Could you check a few things on this model? Use its own coordinates, in mm. Face numbers are marked on the shaded views. A direction names the side the tool comes from. Round coordinates to 2 decimals unless told otherwise and drop trailing zeros. Write each loop counter-clockwise with the first axis right and the second up, starting at its lowest first coordinate (ties: lowest second). Pieces come first, ordered by that corner, then holes. Notation, with made-up numbers: M 3,33 L 23,33 A9 ccw 23,50 Z; hole C 71,12 d11. An arc over 180 degrees is marked long. One line per item, written item: value. Start each with the question number.
(1) If I drill on L1, parallel to X at y = -20, z = 8; L2, parallel to Y at x = 24, z = 6; L3, parallel to X at y = 5, z = 6.5, over which ranges is the centre line in solid material (lowest first)?
(2) Which directions (+Z, -Z, +X, -X, +Y, -Y) give clear straight access to the entire face, cutting with the end or side of a thin tool? Please do the marked faces 5 and 6.
(3) I want a section at B-B on z = 6.5. Please give me the cut outline in (x, y), and give its area (3 significant figures).
(4) I'm going to push a flat-ended pin straight in: pin 1 Ø23.5 at (x, y) = (14, -3) entering from +Z. Where does the tip first touch, or does it pass through?
(5) Thinking about a two-plate mould opening in X: for the marked faces 1, 2, 3 and 4, which applies, released by +X, released by -X, zero draft, split by the parting line, or undercut?
```python
from build123d import *

# Parameters (mm, degrees)
F0_W     = 117.221
F0_H     = 53.721
F1_DEPTH = 19.05
F2_R     = 3.175
F3_T     = -2.54
F5_W     = 11.2527239306
F5_H     = 9.8262102796
F5_W_2   = 11.6953600091
F5_H_2   = 12.192
F6_DEPTH = 17.78


# Not quite as in the source:
# - a feature names something its author has since deleted; it is built from what else it names


with BuildPart() as f1:
    # F0 (on Top) → F1 (new body)
    with BuildSketch(Plane.XY):
        Rectangle(F0_W, F0_H)
    extrude(amount=F1_DEPTH)

    # F2
    f2_edges = [f1.edges().sort_by_distance(p)[0] for p in [
        (0, -26.8605, 0),
        (-58.6105, 0, 0),
        (0, 26.8605, 0),
        (58.6105, 0, 0),
    ]]
    fillet(f2_edges, radius=F2_R)

    # F3
    f3_openings = [f1.faces().sort_by_distance(p)[0] for p in [
        (0, 0, 19.05),
    ]]
    offset(amount=F3_T, openings=f3_openings)

    # F5 (on offset) → F6 (join)
    with BuildSketch(Plane.XY.offset(19.05)):
        with Locations((-51.4034552881, -20.4349435174)):
            Rectangle(F5_W, F5_H)
        with Locations((51.8481470752, 20.1015706725)):
            Rectangle(F5_W_2, F5_H_2)
        with Locations((-51.4034552881, 20.1015706725)):
            Rectangle(F5_W, F5_H_2)
        with Locations((51.8481470752, -20.4349435174)):
            Rectangle(F5_W_2, F5_H)
    extrude(amount=-F6_DEPTH)


solid = f1.part
```
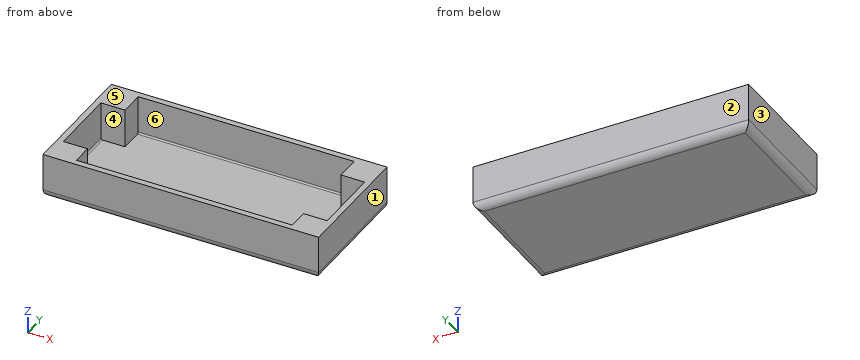
Found:
1. L1: x = -58.61 to -45.78, 46 to 58.61
1. L2: y = -26.86 to -24.32, 24.32 to 26.86
1. L3: x = -58.61 to -56.07, 56.07 to 58.61
2. face 5: +Z, +X, -X, +Y, -Y
2. face 6: +Z
3. outline: M -58.61,-26.86 L 58.61,-26.86 L 58.61,26.86 L -58.61,26.86 Z; hole M -56.07,-15.52 L -45.78,-15.52 L -45.78,-24.32 L 46,-24.32 L 46,-15.52 L 56.07,-15.52 L 56.07,14.01 L 46,14.01 L 46,24.32 L -45.78,24.32 L -45.78,14.01 L -56.07,14.01 Z
3. area: 1,230 mm²
4. pin 1: stops at z = 2.54
5. face 1: released by +X
5. face 2: zero draft
5. face 3: released by -X
5. face 4: undercut
